```python
from build123d import *

# Parameters (mm, degrees)
BOSS_EXTRUDE1_DEPTH     = 10
SKETCH2_R               = 2.6
CUT_EXTRUDE1_DEPTH      = 142.774468788
BOSS_EXTRUDE3_START     = 10
SKETCH3_W               = 60
SKETCH3_H               = 9
SKETCH3_W_2             = 9
SKETCH3_H_2             = 60
BOSS_EXTRUDE3_DEPTH     = 1.46
CUT_EXTRUDE2_DEPTH      = 142.884923794
CUT_EXTRUDE2_DEPTH_BACK = 142.884923794
SKETCH2_2_R             = 2.6
CHAMFER1_SIZE           = 1.46
SKETCH4_R               = 4.5
CUT_EXTRUDE3_DEPTH      = 5
CHAMFER2_SIZE           = 5


with BuildPart() as part:
    # Sketch1 → Boss-Extrude1 (new body)
    with BuildSketch(Plane.XY):
        Polygon((0, 0), (100, 0), (100, 40), (40, 100), (0, 100), align=None)
    extrude(amount=BOSS_EXTRUDE1_DEPTH)

    # Sketch2 → Cut-Extrude1 (cut, through all)
    with BuildSketch(Plane.XY):
        with Locations((10, 85)):
            Circle(SKETCH2_R)
        with Locations((30, 85)):
            Circle(SKETCH2_R)
        with Locations((10, 60)):
            Circle(SKETCH2_R)
        with Locations((30, 60)):
            Circle(SKETCH2_R)
        with Locations((85, 30)):
            Circle(SKETCH2_R)
        with Locations((85, 10)):
            Circle(SKETCH2_R)
        with Locations((60, 10)):
            Circle(SKETCH2_R)
        with Locations((60, 30)):
            Circle(SKETCH2_R)
    extrude(amount=CUT_EXTRUDE1_DEPTH, mode=Mode.SUBTRACT)

    # Sketch3 → Boss-Extrude3 (add)
    with BuildSketch(Plane.XY.offset(BOSS_EXTRUDE3_START)):
        with Locations((70, 30)):
            Rectangle(SKETCH3_W, SKETCH3_H)
        with Locations((70, 10)):
            Rectangle(SKETCH3_W, SKETCH3_H)
        with Locations((10, 70)):
            Rectangle(SKETCH3_W_2, SKETCH3_H_2)
        with Locations((30, 70)):
            Rectangle(SKETCH3_W_2, SKETCH3_H_2)
    extrude(amount=BOSS_EXTRUDE3_DEPTH)

    # Sketch2<2> → Cut-Extrude2 (cut, two sides: drawn at the far end of the back side and taken through both)
    with BuildSketch(Plane.XY.offset(-CUT_EXTRUDE2_DEPTH_BACK)):
        with Locations((10, 85)):
            Circle(SKETCH2_2_R)
        with Locations((30, 85)):
            Circle(SKETCH2_2_R)
        with Locations((10, 60)):
            Circle(SKETCH2_2_R)
        with Locations((30, 60)):
            Circle(SKETCH2_2_R)
        with Locations((85, 30)):
            Circle(SKETCH2_2_R)
        with Locations((85, 10)):
            Circle(SKETCH2_2_R)
        with Locations((60, 10)):
            Circle(SKETCH2_2_R)
        with Locations((60, 30)):
            Circle(SKETCH2_2_R)
    extrude(amount=CUT_EXTRUDE2_DEPTH + CUT_EXTRUDE2_DEPTH_BACK, mode=Mode.SUBTRACT)

    # Chamfer1
    chamfer1_edges = [part.edges().sort_by_distance(p)[0] for p in [
        (14.5, 70, 11.46),
        (5.5, 70, 11.46),
        (25.5, 70, 11.46),
        (34.5, 70, 11.46),
        (70, 5.5, 11.46),
        (70, 14.5, 11.46),
        (70, 25.5, 11.46),
        (70, 34.5, 11.46),
    ]]
    chamfer(chamfer1_edges, length=CHAMFER1_SIZE - 0.0001)  # a hair under: the kernel refuses the full size

    # Sketch4 → Cut-Extrude3 (cut)
    with BuildSketch(Plane.XY):
        with Locations((10, 85)):
            Circle(SKETCH4_R)
        with Locations((30, 85)):
            Circle(SKETCH4_R)
        with Locations((30, 60)):
            Circle(SKETCH4_R)
        with Locations((10, 60)):
            Circle(SKETCH4_R)
        with Locations((60, 30)):
            Circle(SKETCH4_R)
        with Locations((85, 30)):
            Circle(SKETCH4_R)
        with Locations((85, 10)):
            Circle(SKETCH4_R)
        with Locations((60, 10)):
            Circle(SKETCH4_R)
    extrude(amount=CUT_EXTRUDE3_DEPTH, mode=Mode.SUBTRACT)

    # Chamfer2
    chamfer2_edges = [part.edges().sort_by_distance(p)[0] for p in [
        (20, 100, 0),
        (70, 70, 0),
        (100, 20, 0),
        (50, 0, 0),
        (0, 50, 0),
        (0, 100, 5),
        (100, 0, 5),
        (0, 0, 5),
    ]]
    chamfer(chamfer2_edges, length=CHAMFER2_SIZE)


solid = part.part
```
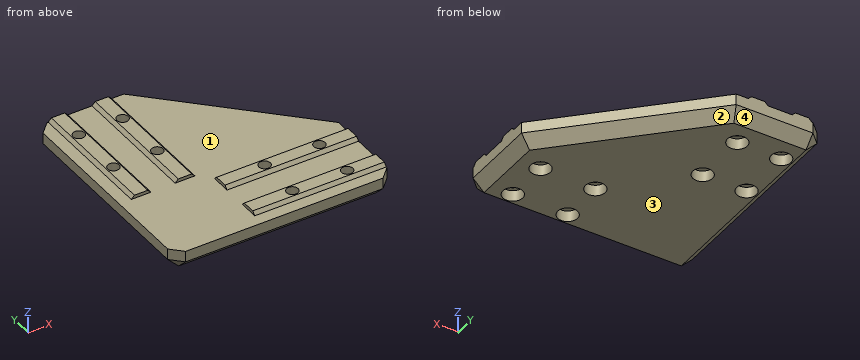
CAD build for the part. Positions are in the model's coordinates, mm. Face numbers are marked on the shaded views. A direction names the side the tool comes from. Coordinates: 2 decimals unless noted, no trailing zeros. Order: outer loops, then holes, each group sorted by start corner. A loop starts at its lowest first (then second) coordinate and runs counter-clockwise, first axis right, second up. Notation, with made-up numbers: (26, 65.25) -> (32, 65.25) arc R10 ccw to (32, 74.25) -> close; hole circle Ø8 at (-29.5, 8). An arc over 180 degrees is marked (long way). Use one line per item in the form item = value. Start each with the question number.
1) Pull direction Y, two halves, no side cores. Call the marked faces 3 and 4: +Y half, -Y half, draft (parallel to the pull), parting line (faces both ways), or undercut.
2) Band-saw the part on C-C on z = 8.75. State how many separate pieces and enclosed holes the cut face has, then the cut area to 3 significant figures.
3) Tool access for the marked faces 1 and 2: list every direction of +Z, -Z, +X, -X, +Y, -Y with a clear straight run to the whole face (end or side of a thin tool).
4) Drill centre lines: L1, parallel to X at y = 10, z = 8.75; L2, parallel to X at y = 86.5, z = 3.25; L3, parallel to Y at x = 85, z = 8.25. Where is each one in solid material? Low to high. Write a range as [from, to].
5) Band-saw the part on A-A on y = 30. Give the cut face in (x, z).
6) Drop flat-ended pins along their axis: pin 1 (1.6 mm diameter, centred on y = 9, z = 10.5, fed in from -X); pin 2 (6 mm diameter, centred on x = 10, y = 60, fed in from -Z); pin 3 (3 mm diameter, centred on x = 85, y = 30, fed in from -Z); pin 4 (5 mm diameter, centred on x = 42.5, z = 3, fed in from +Y). Give the stop position or say it passes through.
Entries:
q1.face_3 = draft
q1.face_4 = +Y half
q2.separate_pieces = 1
q2.enclosed_holes = 8
q2.area = 7,990 mm2
q3.face_1 = +Z
q3.face_2 = -Z, +X, +Y
q4.L1 = [0, 57.4], [62.6, 82.4], [87.6, 100]
q4.L2 = [1.75, 5.76], [14.24, 25.76], [34.24, 51.03]
q4.L3 = [0, 7.4], [12.6, 27.4], [32.6, 55]
q5.outline = (0, 5) -> (5, 0) -> (55.5, 0) -> (55.5, 5) -> (57.4, 5) -> (57.4, 11.46) -> (40, 11.46) -> (40, 10) -> (0, 10) -> close; (62.6, 5) -> (64.5, 5) -> (64.5, 0) -> (80.5, 0) -> (80.5, 5) -> (82.4, 5) -> (82.4, 11.46) -> (62.6, 11.46) -> close; (87.6, 5) -> (89.5, 5) -> (89.5, 0) -> (95, 0) -> (100, 5) -> (100, 11.46) -> (87.6, 11.46) -> close
q6.pin_1 = 0
q6.pin_2 = 5
q6.pin_3 = through
q6.pin_4 = 99
